The model under review builds one solid part; all positions refer to its coordinate system, in mm. Face numbers are marked on the shaded views. A direction names the side the tool comes from. Round coordinates to 2 decimals unless told otherwise and drop trailing zeros. Write each loop counter-clockwise with the first axis right and the second up, starting at its lowest first coordinate (ties: lowest second). Pieces come first, ordered by that corner, then holes. Notation, with made-up numbers: (-37, -37.5) - (-32, -37.5) arc R24 ccw to (-32, -8.5) - close; hole circle Ø9 at (76, 76.5). An arc over 180 degrees is marked (long way). Use one line per item in the form item = value.
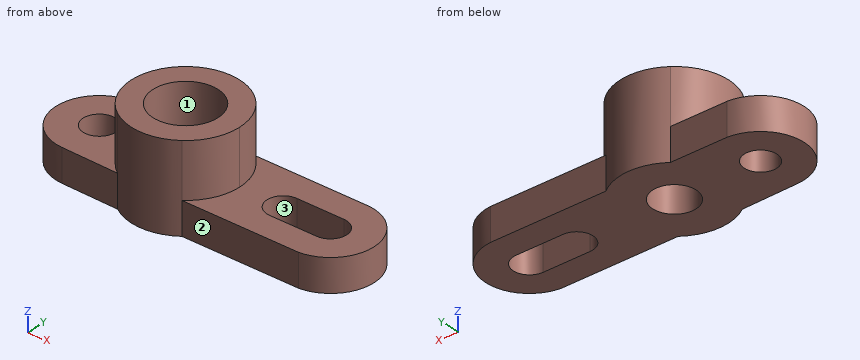
from build123d import *

# Parameters (mm, degrees)
F0_R     = 19.05
F1_DEPTH = 50.8
F0_R_2   = 9.525
F2_DEPTH = 19.05
F0_R_3   = 12.7
F3_DEPTH = 25.4


with BuildPart() as f1:
    # F0 (on Top) → F1 (new body)
    with BuildSketch(Plane.XY):
        with BuildLine():
            ThreePointArc((19.199675, -25.287052), (28.439868, -14.115113), (31.75, 0))
            ThreePointArc((31.75, 0), (28.415813, 14.163477), (19.113523, 25.352234))
            ThreePointArc((19.113523, 25.352234), (0.018633, 31.749995), (-19.083752, 25.374651))
            ThreePointArc((-19.083752, 25.374651), (-31.742751, -0.678404), (-17.982212, -26.166822))
            ThreePointArc((-17.982212, -26.166822), (0.751034, -31.741116), (19.199675, -25.287052))
        make_face()
        Circle(F0_R, mode=Mode.SUBTRACT)
    extrude(amount=F1_DEPTH)

    # F0 (on Top) → F2 (join)
    with BuildSketch(Plane.XY):
        with BuildLine():
            ThreePointArc((-17.982212, -26.166822), (-31.742751, -0.678404), (-19.083752, 25.374651))
            Line((-19.083752, 25.374651), (-49.129671, 25.374651))
            Line((-49.129671, 25.374651), (-52.470329, 25.374651))
            ThreePointArc((-52.470329, 25.374651), (-76.223563, -0.552574), (-51.36625, -25.423262))
            Line((-51.36625, -25.423262), (-17.982212, -26.166822))
        make_face()
        with Locations((-50.8, 0)):
            Circle(F0_R_2, mode=Mode.SUBTRACT)
        with BuildLine():
            ThreePointArc((19.113523, 25.352234), (28.415813, 14.163477), (31.75, 0))
            ThreePointArc((31.75, 0), (28.439868, -14.115113), (19.199675, -25.287052))
            Line((19.199675, -25.287052), (83.205302, -25.287052))
            Line((83.205302, -25.287052), (87.990698, -25.287052))
            ThreePointArc((87.990698, -25.287052), (110.994542, 0.419117), (87.155001, 25.352234))
            Line((87.155001, 25.352234), (84.040999, 25.352234))
            Line((84.040999, 25.352234), (19.113523, 25.352234))
        make_face()
        with BuildLine():
            ThreePointArc((85.471, 9.525), (94.996, -0.000908), (85.469184, -9.525))
            Line((85.469184, -9.525), (57.973988, -9.519757))
            ThreePointArc((57.973988, -9.519757), (48.134291, -0.156846), (57.660339, 9.525))
            Line((57.660339, 9.525), (85.471, 9.525))
        make_face(mode=Mode.SUBTRACT)
    extrude(amount=F2_DEPTH)

    # F0 (on Top) → F3 (join)
    with BuildSketch(Plane.XY):
        Circle(F0_R)
        Circle(F0_R_3, mode=Mode.SUBTRACT)
    extrude(amount=F3_DEPTH)


solid = f1.part
(1) Machinability: for the marked faces 1, 2 and 3, which of the approach directions +Z, -Z, +X, -X, +Y, -Y give a long, thin tool a straight path to every point of the face, cutting with its end or side? Answer none if there is none.
Geometry results:
face_1 = +Z
face_2 = +Z, -Z, +X, -Y
face_3 = +Z, -Z
(2) Add section D-D on x = 60. Write out the cut boundary in (y, z) (3 decimals).
Geometry results:
outline = (-25.287, 0) - (-9.52, 0) - (-9.52, 19.05) - (-25.287, 19.05) - close; (9.525, 0) - (25.352, 0) - (25.352, 19.05) - (9.525, 19.05) - close
(3) Add section B-B on z = 5.5. Write out the cut boundary in (x, y) (3 decimals), then the cut area to 3 significant figures.
Geometry results:
outline = (-52.47, 25.375) arc R25.43 ccw to (-51.366, -25.423) - (-17.982, -26.167) arc R31.75 ccw to (19.2, -25.287) - (87.991, -25.287) arc R25.4 ccw to (87.155, 25.352) - (19.114, 25.352) arc R31.75 ccw to (-19.084, 25.375) - close; hole circle Ø19.05 at (-50.8, 0); hole circle Ø25.4 at (0, 0); hole (57.66, 9.525) arc R9.525 ccw (long way) to (57.974, -9.52) - (85.469, -9.525) arc R9.525 ccw to (85.471, 9.525) - close
area = 7,680 mm2
(4) Add section C-C on z = 41. Write out the cut boundary in (x, y).
Geometry results:
outline = (-19.08, 25.37) arc R31.75 ccw to (-17.98, -26.17) arc R31.75 ccw to (19.2, -25.29) arc R31.75 ccw to (19.11, 25.35) arc R31.75 ccw to start; hole circle Ø38.1 at (0, 0)
(5) To check wall thickness, follow L1, parallel to Y at x = -50.8, z = 4.75 (3 decimals); L2, parallel to Z at x = 84, y = -21.5; L3, parallel to X at y = -4, z = 42.5. State the ranges of each line that lie inside material, in increasing order.
Geometry results:
L1 = -25.436 to -9.525, 9.525 to 25.375
L2 = 0 to 19.05
L3 = -31.5 to -18.63, 18.63 to 31.5
(6) Add section A-A on x = 0. Write out the cut boundary in (y, z).
Geometry results:
outline = (-31.75, 0) - (-12.7, 0) - (-12.7, 25.4) - (-19.05, 25.4) - (-19.05, 50.8) - (-31.75, 50.8) - close; (12.7, 0) - (31.75, 0) - (31.75, 50.8) - (19.05, 50.8) - (19.05, 25.4) - (12.7, 25.4) - close
(7) Insertion check: P1, Ø21, axis at x = -40.5, z = 13, coming from the +Y side; P2, Ø1.5, axis at x = 7.5, z = 25, coming from the +Y side; P3, Ø1.5, axis at x = 27, z = 23.5, coming from the +Y side; P4, Ø5, axis at x = 34, y = -21, coming from the -Z side. Each pin has a flat end and moves straight along its axis. Give the tip position at first contact, or say it passes through.
Geometry results:
P1 = 25.37
P2 = 31.02
P3 = 17.86
P4 = 0
